Part print with two shaded views. Sizes in mm from the minimum x, y, z corner. A direction names the side the tool comes from. Give positions to 0.01 mm unless a question says otherwise; leave off trailing zeros. Write each loop counter-clockwise with the first axis right and the second up, starting at its lowest first coordinate (ties: lowest second). Pieces come first, ordered by that corner, then holes. Notation, with made-up numbers: M 75.25,-22 L 124.25,-22 A22 cw 124.25,2 Z; hole C 18.25,87 d2. An arc over 180 degrees is marked long. Return JSON: item names as keys, results as strings. Group by question number.
Q1. Band-saw the part on C-C, the plane y = 32. Give the cut face in (x, z).
Q2. Tool access for the marked faces 1 and 2: list every direction of +Z, -Z, +X, -X, +Y, -Y with a clear straight run to the whole face (end or side of a thin tool).
Q3. Band-saw the part on D-D, the plane z = 41.5. Give the cut face in (x, y).
Q4. Flat gauge pins, fed straight in: pin 1 Ø10 at (x, y) = (43.5, 5) entering from +Z; pin 2 Ø12 at (x, z) = (24, 36) entering from +Y; pin 3 Ø4 at (x, z) = (35.5, 59) entering from +Y (1 decimal). Where does each tip first touch, or does it go through?
Q5. Band-saw the part on B-B, the plane y = 23. Give the cut face in (x, z), then the cut area to 3 significant figures.
Q6. Wall check: probe 1 along Z at (x, y) = (23.5, 25); probe 2 along Z at (x, y) = (47, 30); probe 3 along Z at (x, y) = (35.5, 24.5). Give the ranges that are in metal, low to high.
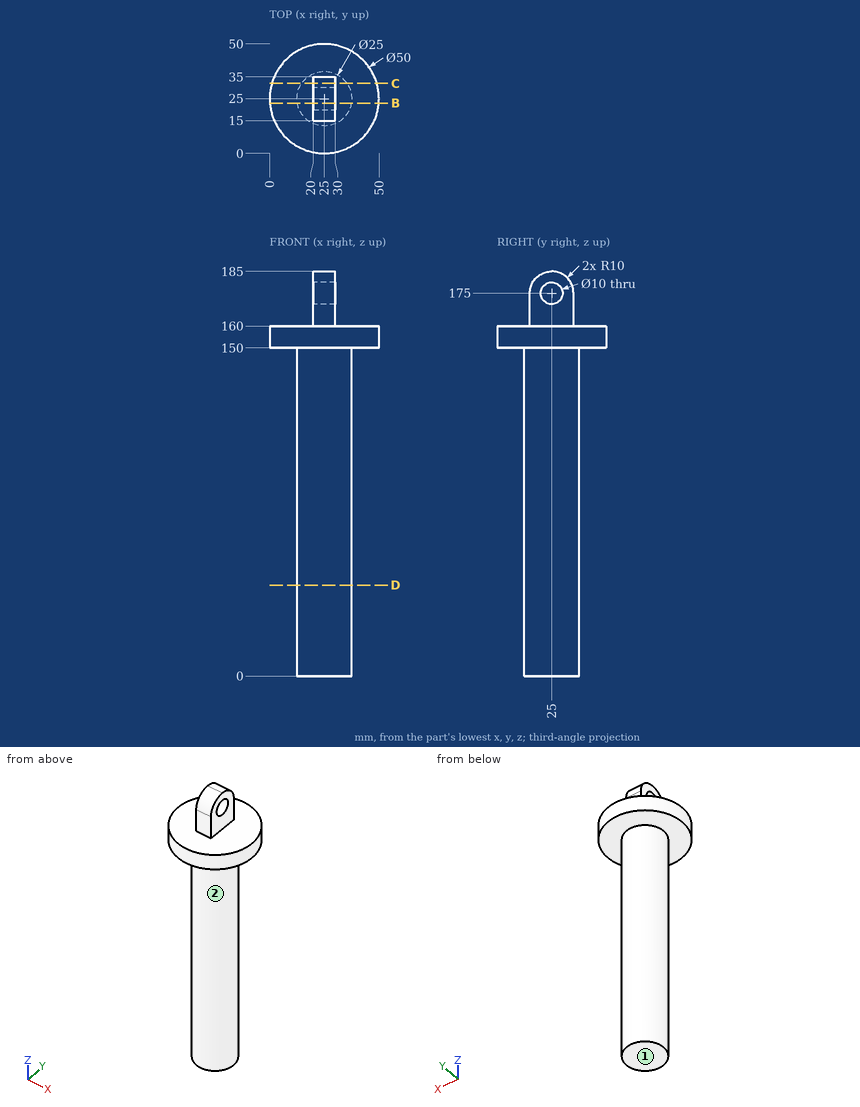
From the geometry:
{
 "1": {"outline": "M 1,150 L 14.64,150 L 14.64,0 L 35.36,0 L 35.36,150 L 49,150 L 49,160 L 30,160 L 30,182.14 L 20,182.14 L 20,160 L 1,160 Z"},
 "2": {"face 1": "-Z, +X, -X, +Y, -Y", "face 2": "-Z"},
 "3": {"outline": "C 25,25 d25"},
 "4": {"pin 1": "stops at z = 160", "pin 2": "stops at y = 37.5", "pin 3": "stops at y = 34.2"},
 "5": {"outline": "M 0.08,150 L 12.66,150 L 12.66,0 L 37.34,0 L 37.34,150 L 49.92,150 L 49.92,160 L 30,160 L 30,170.42 L 20,170.42 L 20,160 L 0.08,160 Z; M 20,179.58 L 30,179.58 L 30,184.8 L 20,184.8 Z", "area": "4,360 mm^2"},
 "6": {"probe 1": "z = 0 to 170, 180 to 185", "probe 2": "z = 150 to 160", "probe 3": "z = 0 to 160"}
}
